```python
from build123d import *

# Parameters (mm, degrees)
F0_R     = 2.25
F1_DEPTH = 3


with BuildPart() as f1:
    # F0 (on Front) → F1 (new body)
    with BuildSketch(Plane.XZ):
        Polygon((-10, -20), (0, -20), (10, -20), (10, -23), (20, -23), (20, -20), (30, -20), (30, -23), (40, -23), (40, -20), (47, -20), (47, -15), (50, -15), (50, -5), (47, -5), (47, 5), (50, 5), (50, 15), (47, 15), (47, 20), (-47, 20), (-47, 15), (-50, 15), (-50, 5), (-47, 5), (-47, -5), (-50, -5), (-50, -15), (-47, -15), (-47, -20), (-40, -20), (-40, -23), (-30, -23), (-30, -20), (-20, -20), (-20, -23), (-10, -23), align=None)
        with Locations((35, 15)):
            Circle(F0_R, mode=Mode.SUBTRACT)
    extrude(amount=F1_DEPTH)


solid = f1.part
```
Part model, mm, in its own coordinate system. A direction names the side the tool comes from. Round coordinates to 2 decimals unless told otherwise and drop trailing zeros. Loops run counter-clockwise (first coordinate to the right, second up) from the corner with the lowest first, then second, coordinate; pieces in that order, holes last.
1. Flat gauge pins, fed straight in: pin 1 (0.9 mm diameter, centred on x = 23, y = -2, fed in from -Z); pin 2 (1.5 mm diameter, centred on x = 49, y = -1, fed in from -Z); pin 3 (1.5 mm diameter, centred on y = -2, z = -22, fed in from -X). Where does each tip first touch, or does it go through?
Solutions:
pin 1: stops at z = -20
pin 2: stops at z = -15
pin 3: stops at x = -40
2. Drill centre lines: line 1 along Z through (x, y) = (35, -0.75); line 2 along X through (y, z) = (-1.3, 1); line 3 along Z through (x, y) = (37, -2.65). Where is each one in solid material? Low to high.
Solutions:
line 1: z = -23 to 12.75, 17.25 to 20
line 2: x = -47 to 47
line 3: z = -23 to 13.97, 16.03 to 20
3. 3-axis set-ups, long thin cutter, end or side, ignore diameter. For faces 5 (the face through (-47, -1, -17)), 6 (the face through (-20, -1, -21)), 7 (the face through (-49, -1, 5)), 8 (the face through (48, -1, -15)): which of +Z, -Z, +X, -X, +Y, -Y reach the whole face in a straight line?
Solutions:
face 5: -Z, -X, +Y, -Y
face 6: -Z, +Y, -Y
face 7: -X, +Y, -Y
face 8: -Z, +X, +Y, -Y
4. Slice it at A-A (x = 35). Give the cut face in (y, z), and give its area (4 significant figures).
Solutions:
outline: (-3, -23) - (0, -23) - (0, 12.75) - (-3, 12.75) - close; (-3, 17.25) - (0, 17.25) - (0, 20) - (-3, 20) - close
area: 115.5 mm2
5. Slice it at B-B (z = 14). Give the cut face in (x, y).
Solutions:
outline: (-50, -3) - (32.98, -3) - (32.98, 0) - (-50, 0) - close; (37.02, -3) - (50, -3) - (50, 0) - (37.02, 0) - close
6. Two-plate mould, pull along X, no slides. Class faces 1 (the face through (47, -1, 0)), 2 (the face through (30, -1, -21)), 3 (the face through (-40, -1, -21)), 4 (the face through (49, -1, -5)): pulls with the +X half, pulls with the -X half, needs draft (parallel to the pull), parting line crosses it, or undercut.
Solutions:
face 1: pulls with the +X half
face 2: undercut
face 3: pulls with the -X half
face 4: needs draft
7. Slice it at C-C (x = 7). Give the cut face in (y, z).
Solutions:
outline: (-3, -20) - (0, -20) - (0, 20) - (-3, 20) - close
